from build123d import *

# Parameters (mm, degrees)
SKETCH5_W            = 10
SKETCH5_H            = 10
BOSS_EXTRUDE6_DEPTH  = 8
CHAMFER10_SIZE       = 3
SKETCH6_W            = 4
SKETCH6_H            = 4
BOSS_EXTRUDE7_DEPTH  = 4
SKETCH7_W            = 10
SKETCH7_H            = 10
BOSS_EXTRUDE9_DEPTH  = 7
CHAMFER13_SIZE       = 3
BOSS_EXTRUDE11_DEPTH = 45


with BuildPart() as part:
    # Sketch5 → Boss-Extrude6 (new body)
    with BuildSketch(Plane(origin=(0, 0, 0), x_dir=(1, 0, 0), z_dir=(0, 1, 0))):
        Rectangle(SKETCH5_W, SKETCH5_H)
    extrude(amount=BOSS_EXTRUDE6_DEPTH)

    # Chamfer10
    chamfer10_edges = [part.edges().sort_by_distance(p)[0] for p in [
        (0, 0, 5),
        (-5, 0, 0),
        (0, 0, -5),
        (5, 0, 0),
    ]]
    chamfer(chamfer10_edges, length=CHAMFER10_SIZE)

    # Sketch6 → Boss-Extrude7 (add)
    with BuildSketch(Plane(origin=(0, 0, 0), x_dir=(1, 0, 0), z_dir=(0, 1, 0))):
        Rectangle(SKETCH6_W, SKETCH6_H)
    extrude(amount=-BOSS_EXTRUDE7_DEPTH)

    # Sketch7 → Boss-Extrude9 (add)
    with BuildSketch(Plane(origin=(0, 8, 0), x_dir=(1, 0, 0), z_dir=(0, 1, 0))):
        Rectangle(SKETCH7_W, SKETCH7_H)
    extrude(amount=BOSS_EXTRUDE9_DEPTH)

    # Chamfer13
    chamfer13_edges = [part.edges().sort_by_distance(p)[0] for p in [
        (-5, 15, 0),
        (0, 15, 5),
        (5, 15, 0),
        (0, 15, -5),
    ]]
    chamfer(chamfer13_edges, length=CHAMFER13_SIZE)

    # Sketch8 → Boss-Extrude11 (add)
    with BuildSketch(Plane(origin=(0, 15, 0), x_dir=(1, 0, 0), z_dir=(0, 1, 0))):
        Polygon((2, 0.828427125), (0.828427125, 2), (-0.828427125, 2), (-2, 0.828427125), (-2, -0.828427125), (-0.828427125, -2), (0.828427125, -2), (2, -0.828427125), align=None)
    extrude(amount=BOSS_EXTRUDE11_DEPTH)


solid = part.part
Here's how the part is built. I have some questions about the finished solid (model axes, mm). A direction names the side the tool comes from. Coordinates: 2 decimals unless noted, no trailing zeros. Order: outer loops, then holes, each group sorted by start corner. A loop starts at its lowest first (then second) coordinate and runs counter-clockwise, first axis right, second up.
Item 1: For faces 1 (the face through (-2, -2, 0)), 2 (the face through (2, -2, 0)), 3 (the face through (1.42, 37.18, -1.41)), 4 (the face through (-1.6, 15, -1.6)), 5 (the face through (-1.42, 37.18, 1.41)), which set-ups out of +Z, -Z, +X, -X, +Y, -Y let a thin tool reach every point of the face, with its end or its side?
Result sheet:
face 1: +Z, -Z, -X, -Y
face 2: +Z, -Z, +X, -Y
face 3: -Z, +X, +Y
face 4: -Z, -X, +Y
face 5: +Z, -X, +Y
Item 2: I need wall thicknesses on line 1 (X direction, y = 26.5, z = -0.5); line 2 (Y direction, x = 1.5, z = -3). Which ranges of each line are inside material? Lowest first, please.
Result sheet:
line 1: x = -2 to 2
line 2: y = 1 to 14
Item 3: If we section it at B-B on x = -3.5: List the corners of the cut face in (y, z) for me.
Result sheet:
outline: (1.5, -3.5) - (3, -5) - (12, -5) - (13.5, -3.5) - (13.5, 3.5) - (12, 5) - (3, 5) - (1.5, 3.5) - close
Item 4: For P1, Ø1.2, axis at x = 0, y = -3, coming from the +Z side; P2, Ø4, axis at x = -3.5, y = 46.5, coming from the -Z side; P3, Ø2, axis at x = 1, y = 27, coming from the -Z side; P4, Ø0.9, axis at x = 1.5, z = -1.5, coming from the +Y side, each with a flat end and sliding along its axis, tell me the tip position at first contact or that it passes through.
Result sheet:
P1: stops at z = 2
P2: stops at z = -1.33
P3: stops at z = -2
P4: stops at y = 60
Item 5: If we section it at A-A on y = 38: List the corners of the cut face in (x, z) for me, plus the area to 3 significant figures.
Result sheet:
outline: (-2, -0.83) - (-0.83, -2) - (0.83, -2) - (2, -0.83) - (2, 0.83) - (0.83, 2) - (-0.83, 2) - (-2, 0.83) - close
area: 13.3 mm2
